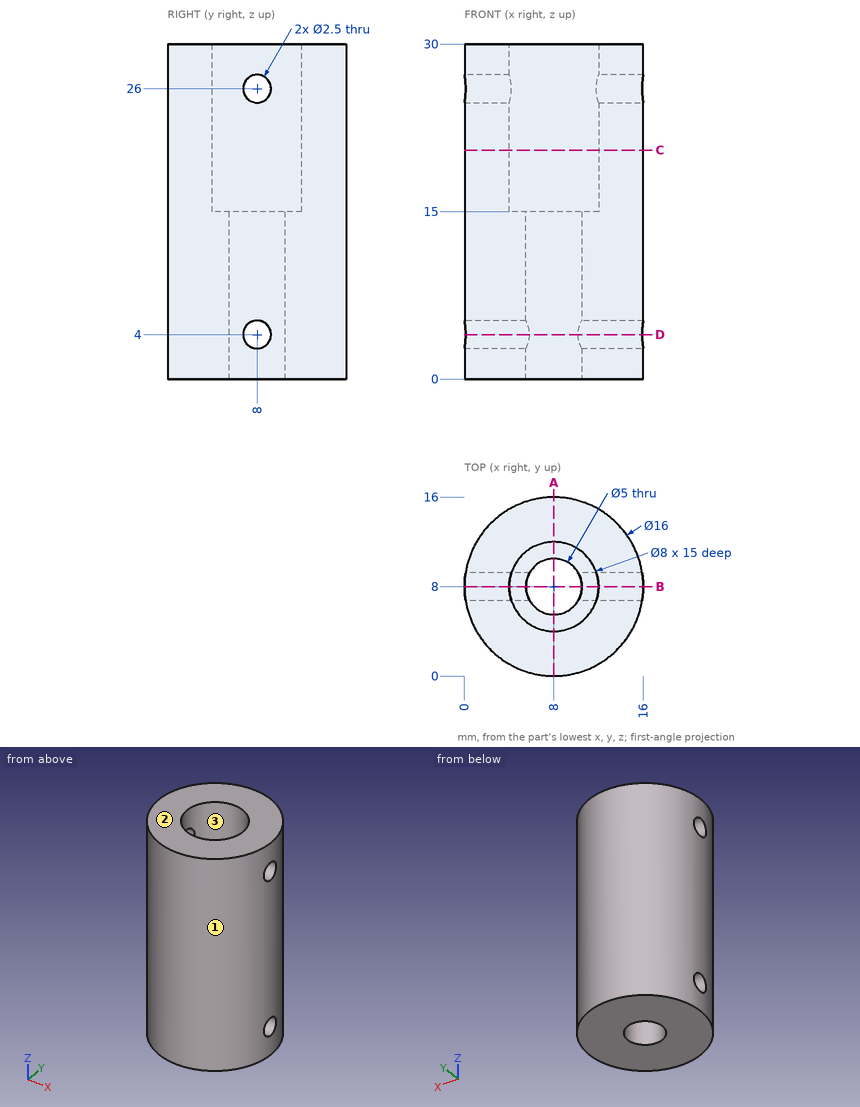
Input: dimensioned drawing with shaded views. Units: mm. Origin: part minimum x, y, z. Give positions to 0.01 mm unless a question says otherwise; leave off trailing zeros. Order: outer loops, then holes, each group sorted by start corner. A loop starts at its lowest first (then second) coordinate and runs counter-clockwise, first axis right, second up.
(1) Section query D-D (z = 4). Return the cut outline in (x, y).
(2) Material intervals for line 1 along Y through (x, z) = (8, 28); line 2 along Y through (x, z) = (6, 10); line 3 along X through (y, z) = (11.25, 27), sorted ascending.
(3) Section query B-B (y = 8). Return the cut outline in (x, z), plus the area to 4 significant figures.
(4) Section query C-C (z = 20.5). Return the cut outline in (x, y), plus the area to 3 significant figures.
(5) Section query A-A (x = 8). Return the cut outline in (y, z).
(6) Pull-direction query (X, two-part tool) for the marked faces 1, 2 and 3; classes: +X half, -X half, draft (parallel to the pull), parting line (faces both ways), or undercut.
(7) Contact query for flat-ended pins moving along their axis: P1, Ø6, axis at x = 8, y = 8, coming from the +Z side; P2, Ø2, axis at y = 8, z = 4, coming from the -X side; P3, Ø6, axis at x = 12.5, z = 5.5, coming from the -Y side; P4, Ø3, axis at x = 3, z = 12.5, coming from the +Y side. Output: stop coordinate, or through.
Outcome:
1. outline: (0.1, 6.75) arc R8 ccw to (15.9, 6.75) - (10.17, 6.75) arc R2.5 cw to (5.83, 6.75) - close; (0.1, 9.25) - (5.83, 9.25) arc R2.5 cw to (10.17, 9.25) - (15.9, 9.25) arc R8 ccw to start
2. line 1: y = 0 to 4, 12 to 16
2. line 2: y = 0.25 to 6.5, 9.5 to 15.75
2. line 3: x = 0.69 to 5.67, 10.33 to 15.31
3. outline: (0, 0) - (5.5, 0) - (5.5, 2.75) - (0, 2.75) - close; (0, 5.25) - (5.5, 5.25) - (5.5, 15) - (4, 15) - (4, 24.75) - (0, 24.75) - close; (0, 27.25) - (4, 27.25) - (4, 30) - (0, 30) - close; (10.5, 0) - (16, 0) - (16, 2.75) - (10.5, 2.75) - close; (10.5, 5.25) - (16, 5.25) - (16, 24.75) - (12, 24.75) - (12, 15) - (10.5, 15) - close; (12, 27.25) - (16, 27.25) - (16, 30) - (12, 30) - close
3. area: 237.5 mm2
4. outline: circle Ø16 at (8, 8); hole circle Ø8 at (8, 8)
4. area: 151 mm2
5. outline: (0, 0) - (5.5, 0) - (5.5, 15) - (4, 15) - (4, 30) - (0, 30) - close; (10.5, 0) - (16, 0) - (16, 30) - (12, 30) - (12, 15) - (10.5, 15) - close
6. face 1: parting line
6. face 2: draft
6. face 3: undercut
7. P1: stops at z = 15
7. P2: passes through
7. P3: stops at y = 0.14
7. P4: stops at y = 15.19
